Can you work these out from the model? Positions are in its coordinate system, mm. Face numbers are marked on the shaded views. A direction names the side the tool comes from. Coordinates: 2 decimals unless noted, no trailing zeros. Order: outer loops, then holes, each group sorted by start corner. A loop starts at its lowest first (then second) coordinate and runs counter-clockwise, first axis right, second up. Notation, with made-up numbers: (-13, 26) -> (7, 26) arc R28 ccw to (7, 62) -> close; hole circle Ø1 at (-37.75, 88.25). An arc over 180 degrees is marked (long way). Answer in a Markdown table with one row per item.
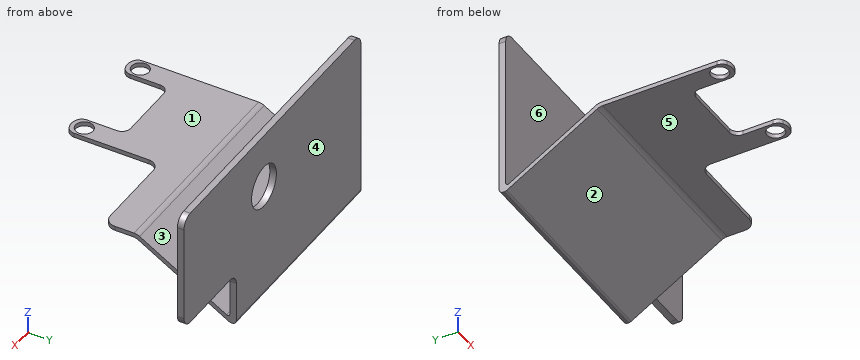
```python
from build123d import *

# Parameters (mm, degrees)
SKETCH1_R           = 4.896847049
BOSS_EXTRUDE1_DEPTH = 1.5
BOSS_EXTRUDE4_DEPTH = 49
FILLET1_R           = 1
FILLET2_R           = 0.5
SKETCH3_R           = 2
BOSS_EXTRUDE6_DEPTH = 1
FILLET3_R           = 2.5
FILLET4_R           = 2.5


with BuildPart() as part:
    # Sketch1 → Boss-Extrude1 (new body)
    with BuildSketch(Plane(origin=(0, 0, 0), x_dir=(1, 0, 0), z_dir=(0, 1, 0))):
        with BuildLine():
            Line((-32.322023461, -13.602352914), (32.322023461, -13.602352914))
            ThreePointArc((32.322023461, -13.602352914), (34.089790414, -12.870119867), (34.822023461, -11.102352914))
            Line((34.822023461, -11.102352914), (34.822023461, 11.102352914))
            ThreePointArc((34.822023461, 11.102352914), (34.089790414, 12.870119867), (32.322023461, 13.602352914))
            Line((32.322023461, 13.602352914), (16.677976539, 13.602352914))
            ThreePointArc((16.677976539, 13.602352914), (14.910209586, 14.334585961), (14.177976539, 16.102352914))
            Line((14.177976539, 16.102352914), (14.177976539, 26.397647086))
            Line((14.177976539, 26.397647086), (-32.322023461, 26.397647086))
            Line((-32.322023461, 26.397647086), (-34.822023461, 26.397647086))
            Line((-34.822023461, 26.397647086), (-34.822023461, 23.897647086))
            Line((-34.822023461, 23.897647086), (-34.822023461, 13.602352914))
            Line((-34.822023461, 13.602352914), (-34.822023461, -11.102352914))
            Line((-34.822023461, -11.102352914), (-34.822023461, -13.602352914))
            Line((-34.822023461, -13.602352914), (-32.322023461, -13.602352914))
        make_face()
        with Locations(Location((3.322023461, -0.897647086, 0), (0, 0, 270))):
            Circle(SKETCH1_R, mode=Mode.SUBTRACT)
    extrude(amount=BOSS_EXTRUDE1_DEPTH)

    # Sketch2 → Boss-Extrude4 (add)
    with BuildSketch(Plane(origin=(14.177976539, 0, 0), x_dir=(0, 0, -1), z_dir=(1, 0, 0))):
        with BuildLine():
            Line((25.233954828, 0), (12.954018608, -20.634041328))
            ThreePointArc((12.954018608, -20.634041328), (12.691872074, -21.249569549), (12.602352914, -21.912579441))
            Line((12.602352914, -21.912579441), (12.602352914, -28.802677945))
            Line((12.602352914, -28.802677945), (13.602352914, -28.802677945))
            Line((13.602352914, -28.802677945), (13.602352914, -22.187632402))
            ThreePointArc((13.602352914, -22.187632402), (13.691872074, -21.52462251), (13.954018608, -20.909094288))
            Line((13.954018608, -20.909094288), (26.397647086, 0))
            Line((26.397647086, 0), (25.233954828, 0))
        make_face()
    extrude(amount=-BOSS_EXTRUDE4_DEPTH)

    # Fillet1
    fillet1_edges = [part.edges().sort_by_distance(p)[0] for p in [
        (-10.322023461, 0, -26.397647086),
        (-10.322023461, 1.5, -26.397647086),
    ]]
    fillet(fillet1_edges, radius=FILLET1_R)

    # Fillet2
    fillet2_edges = [part.edges().sort_by_distance(p)[0] for p in [
        (-10.322023461, 0, -25.233954828),
    ]]
    fillet(fillet2_edges, radius=FILLET2_R)

    # Sketch3 → Boss-Extrude6 (add)
    with BuildSketch(Plane.XY.offset(-12.602352914)):
        with BuildLine():
            Line((-27.822023461, -39.5), (-14.772023461, -39.5))
            ThreePointArc((-14.772023461, -39.5), (-13.357809898, -40.085786438), (-12.772023461, -41.5))
            Line((-12.772023461, -41.5), (-12.772023461, -48.366025404))
            ThreePointArc((-12.772023461, -48.366025404), (-12.504074268, -49.366025404), (-11.772023461, -50.098076211))
            ThreePointArc((-11.772023461, -50.098076211), (-10.272023461, -50.5), (-8.772023461, -50.098076211))
            ThreePointArc((-8.772023461, -50.098076211), (-8.039972653, -49.366025404), (-7.772023461, -48.366025404))
            Line((-7.772023461, -48.366025404), (-7.772023461, -39.5))
            Line((-7.772023461, -39.5), (-7.772023461, -28.802677945))
            Line((-7.772023461, -28.802677945), (-34.822023461, -28.802677945))
            Line((-34.822023461, -28.802677945), (-34.822023461, -39.5))
            Line((-34.822023461, -39.5), (-34.822023461, -48.366025404))
            ThreePointArc((-34.822023461, -48.366025404), (-34.554074268, -49.366025404), (-33.822023461, -50.098076211))
            ThreePointArc((-33.822023461, -50.098076211), (-32.322023461, -50.5), (-30.822023461, -50.098076211))
            ThreePointArc((-30.822023461, -50.098076211), (-30.089972653, -49.366025404), (-29.822023461, -48.366025404))
            Line((-29.822023461, -48.366025404), (-29.822023461, -41.5))
            ThreePointArc((-29.822023461, -41.5), (-29.236237023, -40.085786438), (-27.822023461, -39.5))
        make_face()
        with Locations((-32.322023461, -47.5)):
            Circle(SKETCH3_R, mode=Mode.SUBTRACT)
        with Locations((-10.272023461, -47.5)):
            Circle(SKETCH3_R, mode=Mode.SUBTRACT)
    extrude(amount=-BOSS_EXTRUDE6_DEPTH)

    # Fillet3
    fillet3_edges = [part.edges().sort_by_distance(p)[0] for p in [
        (14.177976539, -28.802677945, -13.102352914),
        (-7.772023461, -28.802677945, -13.102352914),
    ]]
    fillet(fillet3_edges, radius=FILLET3_R)

    # Fillet4
    fillet4_edges = [part.edges().sort_by_distance(p)[0] for p in [
        (-34.822023461, 0.75, 13.602352914),
    ]]
    fillet(fillet4_edges, radius=FILLET4_R)


solid = part.part
```
(1) Will these pins go through, and if not, where does the flat tip stop? pin 1 Ø8 at (y, z) = (-22.5, -5.5) entering from -X; pin 2 Ø5 at (x, y) = (-32.32, -47.5) entering from +Z; pin 3 Ø0.8 at (x, z) = (0, -13) entering from -Y; pin 4 Ø1.2 at (x, y) = (21.5, 0.5) entering from -Z.
Response values:
| item | result |
|---|---|
| pin 1 | through |
| pin 2 | z = -12.6 |
| pin 3 | y = -28.8 |
| pin 4 | z = -13.6 |
(2) Suppose I cut it at A-A (y = -47.5). Please give me the cut outline in (x, z).
Response values:
| item | result |
|---|---|
| outline | (-34.82, -13.6) -> (-34.32, -13.6) -> (-34.32, -12.6) -> (-34.82, -12.6) -> close; (-30.32, -13.6) -> (-29.82, -13.6) -> (-29.82, -12.6) -> (-30.32, -12.6) -> close; (-12.77, -13.6) -> (-12.27, -13.6) -> (-12.27, -12.6) -> (-12.77, -12.6) -> close; (-8.27, -13.6) -> (-7.77, -13.6) -> (-7.77, -12.6) -> (-8.27, -12.6) -> close |
(3) Suppose I cut it at B-B (z = 2.5). Please give me the cut outline in (x, y).
Response values:
| item | result |
|---|---|
| outline | (-34.82, 0) -> (-1.31, 0) -> (-1.31, 1.5) -> (-34.82, 1.5) -> close; (7.95, 0) -> (34.82, 0) -> (34.82, 1.5) -> (7.95, 1.5) -> close |
(4) I need wall thicknesses on line 1 (Y direction, x = -21, z = -1.5); line 2 (Y direction, x = -31, z = -13); line 3 (Z direction, x = -18.5, y = -37.5). Which ranges of each line are inside material? Lowest first, please. Write a range as [from, to].
Response values:
| item | result |
|---|---|
| line 1 | [0, 1.5] |
| line 2 | [-50.19, -49], [-46, -20.56], [0, 1.5] |
| line 3 | [-13.6, -12.6] |
(5) We'd pull the mould along Y, two halves only. Please class the marked faces 4, 5 and 6: +Y half, -Y half, draft (parallel to the pull), parting line (faces both ways), or undercut.
Response values:
| item | result |
|---|---|
| face 4 | +Y half |
| face 5 | draft |
| face 6 | undercut |
(6) On a 3-axis mill with a long thin cutter (end or side, diameter ignored), from which of +Z, -Z, +X, -X, +Y, -Y can I reach the whole of each face in a straight line? I mean the marked faces 1, 2 and 3. Say none if no direction works.
Response values:
| item | result |
|---|---|
| face 1 | +Z, +X, -X, -Y |
| face 2 | -Z, +X, -X, -Y |
| face 3 | +Z, +X, -X |
(7) Suppose I cut it at C-C (x = 0). Please give me the cut outline in (y, z), and give its area (3 significant figures).
Response values:
| item | result |
|---|---|
| outline | (-28.8, -13.6) -> (-22.19, -13.6) arc R2.5 cw to (-20.91, -13.95) -> (-0.24, -26.26) arc R1 ccw to (0.28, -26.4) -> (0.5, -26.4) arc R1 ccw to (1.5, -25.4) -> (1.5, -2.7) -> (0, -2.7) -> (0, -24.35) arc R0.5 cw to (-0.76, -24.78) -> (-20.63, -12.95) arc R2.5 ccw to (-21.91, -12.6) -> (-28.8, -12.6) -> close; (0, 4.5) -> (1.5, 4.5) -> (1.5, 13.6) -> (0, 13.6) -> close |
| area | 81.5 mm2 |
(8) Suppose I cut it at D-D (x = 26). Please give me the cut outline in (y, z).
Response values:
| item | result |
|---|---|
| outline | (0, -13.6) -> (1.5, -13.6) -> (1.5, 13.6) -> (0, 13.6) -> close |
